Verification items for the finished model (mm, model axes). Face numbers are marked on the shaded views. A direction names the side the tool comes from. Give positions to 0.01 mm unless a question says otherwise; leave off trailing zeros. Write each loop counter-clockwise with the first axis right and the second up, starting at its lowest first coordinate (ties: lowest second). Pieces come first, ordered by that corner, then holes. Notation, with made-up numbers: M 32.5,49 L 55.5,49 A14 cw 55.5,54 Z; hole C 72.25,61 d2. An arc over 180 degrees is marked long. Write item = value, one per line.
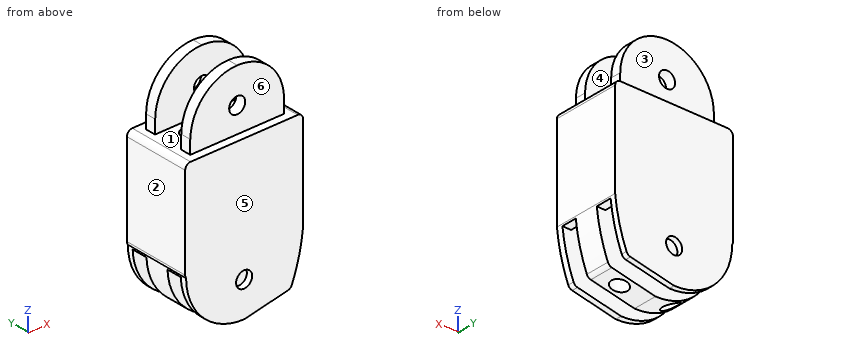
from build123d import *

# Parameters (mm, degrees)
SKETCH2_W               = 17.554431489
SKETCH2_H               = 1.95
BOSS_EXTRUDE1_DEPTH     = 8.75
BOSS_EXTRUDE1_2_DEPTH   = 8.75
CUT_EXTRUDE1_DEPTH      = 26.518349076
SKETCH4_W               = 22.027215745
SKETCH4_H               = 12.505427167
BOSS_EXTRUDE2_DEPTH     = 32
SKETCH5_R               = 1.5
CUT_EXTRUDE2_DEPTH      = 12
SKETCH6_W               = 22.027215745
SKETCH6_H               = 12.505427167
SKETCH6_W_2             = 17.554431489
SKETCH6_H_2             = 1.95
CUT_EXTRUDE3_DEPTH      = 2.5
SKETCH7_R               = 1.5
CUT_EXTRUDE4_DEPTH      = 13
CUT_EXTRUDE5_DEPTH      = 10
CUT_EXTRUDE5_DEPTH_BACK = 32
SKETCH8_R               = 1.5
FILLET3_R               = 1
SKETCH9_W               = 22.034876082
SKETCH9_H               = 2.976325088
SKETCH9_H_2             = 2.861616895
CUT_EXTRUDE6_DEPTH      = 11
SKETCH10_W              = 17.922244656
SKETCH10_H              = 2.976325088
SKETCH10_H_2            = 2.861616895
CUT_EXTRUDE7_DEPTH      = 5


with BuildPart() as part:
    # Sketch2 → Boss-Extrude1 (new body)
    with BuildSketch(Plane.XY):
        with Locations((-13.228930986, -27.845183414)):
            Rectangle(SKETCH2_W, SKETCH2_H)
    extrude(amount=BOSS_EXTRUDE1_DEPTH)


with BuildPart() as body_2:
    # Sketch2 → Boss-Extrude1 2 (new body)
    with BuildSketch(Plane.XY):
        with Locations((-13.228930986, -20.289756247)):
            Rectangle(SKETCH2_W, SKETCH2_H)
    extrude(amount=BOSS_EXTRUDE1_2_DEPTH)


with BuildPart() as cut_extrude1_tool:
    # Sketch3 → Cut-Extrude1 (new, through all)
    with BuildSketch(Plane(origin=(0, -19.314756247, 0), x_dir=(1, 0, 0), z_dir=(0, 1, 0))):
        with BuildLine():
            ThreePointArc((-13.228930986, -8.75), (-7.041746651, -6.187184335), (-4.478930986, 0))
            add(Edge.make_bspline(
                [(-4.478930986, 0), (1.138349918, -4.151657709), (-4.451715242, -8.75)],
                knots=[0, 0, 0, 1, 1, 1], degree=2))
            add(Edge.make_bspline(
                [(-22.006146731, -8.75), (-13.228930986, -12.473510392), (-4.451715242, -8.75)],
                knots=[0, 0, 0, 1, 1, 1], degree=2))
            add(Edge.make_bspline(
                [(-21.978930986, 0), (-25.926969228, -4.242865138), (-22.006146731, -8.75)],
                knots=[0, 0, 0, 1, 1, 1], degree=2))
            ThreePointArc((-21.978930986, 0), (-19.416115322, -6.187184335), (-13.228930986, -8.75))
        make_face()
    extrude(amount=-CUT_EXTRUDE1_DEPTH)


with BuildPart() as part_1:
    add(part.part)

    # Cut-Extrude1: cut by cut_extrude1_tool
    add(cut_extrude1_tool.part, mode=Mode.SUBTRACT)



with BuildPart() as body_2_1:
    add(body_2.part)

    # Cut-Extrude1: cut by cut_extrude1_tool
    add(cut_extrude1_tool.part, mode=Mode.SUBTRACT)


with BuildPart() as part_2:
    add(part_1.part)

    add(body_2_1.part)  # Boss-Extrude2 merges body 2
    # Sketch4 → Boss-Extrude2 (add)
    with BuildSketch(Plane(origin=(0, 0, 0), x_dir=(-1, 0, 0), z_dir=(0, 0, -1))):
        with Locations((13.242538859, -24.067469831)):
            Rectangle(SKETCH4_W, SKETCH4_H)
    extrude(amount=BOSS_EXTRUDE2_DEPTH)

    # Sketch5 → Cut-Extrude2 (cut)
    with BuildSketch(Plane(origin=(0, -19.314756247, 0), x_dir=(1, 0, 0), z_dir=(0, 1, 0))):
        with Locations(Location((-13.228930986, -2.25, 0), (0, 0, 270))):
            Circle(SKETCH5_R)
    extrude(amount=-CUT_EXTRUDE2_DEPTH, mode=Mode.SUBTRACT)

    # Sketch6 → Cut-Extrude3 (cut)
    with BuildSketch(Plane.XY):
        with Locations((-13.242538859, -24.067469831)):
            Rectangle(SKETCH6_W, SKETCH6_H)
        with Locations((-13.228930986, -27.845183414)):
            Rectangle(SKETCH6_W_2, SKETCH6_H_2, mode=Mode.SUBTRACT)
        with Locations((-13.228930986, -20.289756247)):
            Rectangle(SKETCH6_W_2, SKETCH6_H_2, mode=Mode.SUBTRACT)
    extrude(amount=-CUT_EXTRUDE3_DEPTH, mode=Mode.SUBTRACT)

    # Sketch7 → Cut-Extrude4 (cut)
    with BuildSketch(Plane(origin=(0, -17.814756247, 0), x_dir=(1, 0, 0), z_dir=(0, 1, 0))):
        with Locations(Location((-13.242538859, 25.5, 0), (0, 0, 270))):
            Circle(SKETCH7_R)
        with BuildLine():
            Line((-24.086865874, 21.155672985), (-24.256146731, 21.155672985))
            add(Edge.make_bspline(
                [(-2.228930986, 21.155672985), (11.471530889, 27.189710441), (-11.765166974, 53.431279988), (-37.007876173, 21.523583672), (-24.256146731, 21.155672985)],
                knots=[0, 0, 0, 0, 0.52011282, 1, 1, 1, 1], degree=3))
            add(Edge.make_bspline(
                [(-4.552660132, 30.311399113), (-2.685211009, 25.928521854), (-2.228930986, 21.155672985)],
                knots=[0, 0, 0, 1, 1, 1], degree=2))
            Line((-4.552660132, 30.311399113), (-13.242538859, 32))
            ThreePointArc((-13.242538859, 32), (-20.910636028, 28.823770155), (-24.086865874, 21.155672985))
        make_face()
    extrude(amount=-CUT_EXTRUDE4_DEPTH, mode=Mode.SUBTRACT)

    # Sketch8 → Cut-Extrude5 (cut, two sides: drawn at the far end of the back side and taken through both)
    with BuildSketch(Plane.XY.offset(-2.5).offset(-CUT_EXTRUDE5_DEPTH_BACK)):
        with Locations(Location((-18.011106811, -24.06746983, 0), (0, 0, 180))):
            Circle(SKETCH8_R)
        with Locations(Location((-8.473970906, -24.06746983, 0), (0, 0, 180))):
            Circle(SKETCH8_R)
    extrude(amount=CUT_EXTRUDE5_DEPTH + CUT_EXTRUDE5_DEPTH_BACK, mode=Mode.SUBTRACT)

    # Fillet3
    # the kernel refuses this fillet: 1 mm, written as the material it takes off along each edge
    with BuildSketch(Plane(origin=(-24.256146731, -15.314756247, -2.5), x_dir=(0, 0, -1), z_dir=(0, -1, 0)), Plane(origin=(-2.228930986, -32.820183414, -2.5), x_dir=(0, 0, -1), z_dir=(0, 1, 0))) as fillet3_piece_1:
        with BuildLine():
            CenterArc((FILLET3_R, FILLET3_R), FILLET3_R, 180, 90)
            Line((0, FILLET3_R), (-FILLET3_R * 0.02, FILLET3_R))
            Line((-FILLET3_R * 0.02, FILLET3_R), (-FILLET3_R * 0.02, -FILLET3_R * 0.02))
            Line((-FILLET3_R * 0.02, -FILLET3_R * 0.02), (FILLET3_R, -FILLET3_R * 0.02))
            Line((FILLET3_R, -FILLET3_R * 0.02), (FILLET3_R, 0))
        make_face()
    extrude(amount=17.505427167, mode=Mode.SUBTRACT)
    with BuildSketch(Plane(origin=(-24.256146731, -16.423026869, -21.155672985), x_dir=(1.0, 0, 2.5394386720559264e-12), z_dir=(0, -1, 0))) as fillet3_piece_2:
        with BuildLine():
            CenterArc((1, 0.556691751), FILLET3_R, 180, 33.827317624)
            Line((0, 0.556691751), (-0.02, 0.556691751))
            Line((-0.02, 0.556691751), (-0.02, 0))
            Line((-0.02, 0), (0, -0.02))
            ThreePointArc((0, -0.02), (0.084640429, -0.02), (0.152666474, -0.011133835))
            Line((0.152666474, -0.011133835), (0.169280857, 0))
        make_face()
    extrude(amount=15.288885922, mode=Mode.SUBTRACT)
    with BuildSketch(Plane(origin=(-4.552660132, -16.451585564, -30.311399113), x_dir=(0.3839298520349852, 0, 0.9233622629912891), z_dir=(0, -1, 0))) as fillet3_piece_3:
        with BuildLine():
            CenterArc((0.536514164, 0.999961682), FILLET3_R, 213.573886674, 56.927693277)
            Line((-0.296659206, 0.446949805), (-0.313322674, 0.435889568))
            Line((-0.313322674, 0.435889568), (-0.016663467, -0.011060238))
            Line((-0.016663467, -0.011060238), (-0.0001747, -0.019999237))
            ThreePointArc((-0.0001747, -0.019999237), (0.272634035, -0.021192075), (0.545443356, -0.019999234))
            Line((0.545443356, -0.019999234), (0.545268273, 0))
        make_face()
    extrude(amount=15.231768533, mode=Mode.SUBTRACT)

    # Sketch9 → Cut-Extrude6 (cut)
    with BuildSketch(Plane.XY.offset(-32.5)):
        with Locations((-13.229542087, -20.326593706)):
            Rectangle(SKETCH9_W, SKETCH9_H)
        with Locations((-13.229542087, -27.750991873)):
            Rectangle(SKETCH9_W, SKETCH9_H_2)
    extrude(amount=CUT_EXTRUDE6_DEPTH, mode=Mode.SUBTRACT)

    # Sketch10 → Cut-Extrude7 (cut)
    with BuildSketch(Plane(origin=(0, 0, -21.5), x_dir=(-1, 0, 0), z_dir=(0, 0, -1))):
        with Locations((12.848616278, -20.326593706)):
            Rectangle(SKETCH10_W, SKETCH10_H)
        with Locations((12.848616278, -27.750991873)):
            Rectangle(SKETCH10_W, SKETCH10_H_2)
    extrude(amount=-CUT_EXTRUDE7_DEPTH, mode=Mode.SUBTRACT)


solid = part_2.part
1) Cross-section at B-B on x = -9. Record the boundary of the cut face in (y, z), plus the area to 3 significant figures.
From the geometry:
outline = M -30.32,-31.18 L -29.18,-31.18 L -29.18,-16.5 L -26.32,-16.5 L -26.32,-31.18 L -25.47,-31.18 L -25.47,-2.5 L -26.87,-2.5 L -26.87,7.66 L -28.82,7.66 L -28.82,-2.5 L -30.32,-2.5 Z; M -22.66,-31.18 L -21.81,-31.18 L -21.81,-16.5 L -18.84,-16.5 L -18.84,-31.18 L -17.81,-31.18 L -17.81,-2.5 L -19.31,-2.5 L -19.31,7.66 L -21.26,7.66 L -21.26,-2.5 L -22.66,-2.5 Z
area = 232 mm^2
2) Cross-section at D-D on x = -18.75. Record the boundary of the cut face in (y, z).
From the geometry:
outline = M -30.32,-30.5 L -29.18,-30.5 L -29.18,-16.5 L -26.32,-16.5 L -26.32,-30.5 L -25.37,-30.5 L -25.37,-2.5 L -26.87,-2.5 L -26.87,6.79 L -28.82,6.79 L -28.82,-2.5 L -30.32,-2.5 Z; M -22.76,-30.5 L -21.81,-30.5 L -21.81,-16.5 L -18.84,-16.5 L -18.84,-30.5 L -17.81,-30.5 L -17.81,-2.5 L -19.31,-2.5 L -19.31,6.79 L -21.26,6.79 L -21.26,-2.5 L -22.76,-2.5 Z
3) Tool access check on the marked faces 4, 5 and 6. Record the directions out of +Z, -Z, +X, -X, +Y, -Y that give a thin tool (end or side, any length) a straight path to the whole face; none if there is none.
From the geometry:
face_4 = +Z, +X, -X
face_5 = +Z, -Z, +X, -X, -Y
face_6 = +Z, +X, -X, -Y
4) Cross-section at A-A on z = -1. Record the boundary of the cut face in (x, y).
From the geometry:
outline = M -22.01,-28.82 L -4.45,-28.82 L -4.45,-26.87 L -22.01,-26.87 Z; M -22.01,-21.26 L -4.45,-21.26 L -4.45,-19.31 L -22.01,-19.31 Z
5) Draft check along Y on the marked faces 1, 2 and 3. Enter one of: +Y half, -Y half, draft (parallel to the pull), parting line (faces both ways), or undercut.
From the geometry:
face_1 = undercut
face_2 = draft
face_3 = +Y half
6) Material ranges on probe 1 along Y at (x, z) = (-20.5, -19); probe 2 along X at (y, z) = (-23.75, -26); probe 3 along X at (y, z) = (-23.3, -25.5), recorded low to high. Write a range as from..to.
From the geometry:
probe_1 = -30.32..-29.18, -26.32..-21.81, -18.84..-17.81
probe_2 = -22.94..-19.48, -16.55..-14.66, -11.83..-9.94, -7.01..-3.08
probe_3 = -23.18..-19.3, -16.72..-14.74, -11.74..-9.76, -7.19..-2.96
7) Depth check by flat-ended pin: P1, Ø1.5, axis at x = -19.5, y = -25, coming from the -Z side; P2, Ø0.5, axis at x = -3, y = -20, coming from the -Z side; P3, Ø1.5, axis at x = -14, y = -19.5, coming from the -Z side. Enter the tip coordinate at first touch or a pass-through.
From the geometry:
P1 = -30.45
P2 = -21.5
P3 = -31.99
8) Cross-section at C-C on y = -23.5. Count the separate pieces of the cut face and the enclosed holes in it, plus the area to 3 significant figures.
From the geometry:
separate_pieces = 3
enclosed_holes = 1
area = 437 mm^2
